Could you check a few things on this drawing? It's one solid part, dimensions in mm from its lowest x, y, z. A direction names the side the tool comes from. Coordinates: 2 decimals unless noted, no trailing zeros. Order: outer loops, then holes, each group sorted by start corner. A loop starts at its lowest first (then second) coordinate and runs counter-clockwise, first axis right, second up.
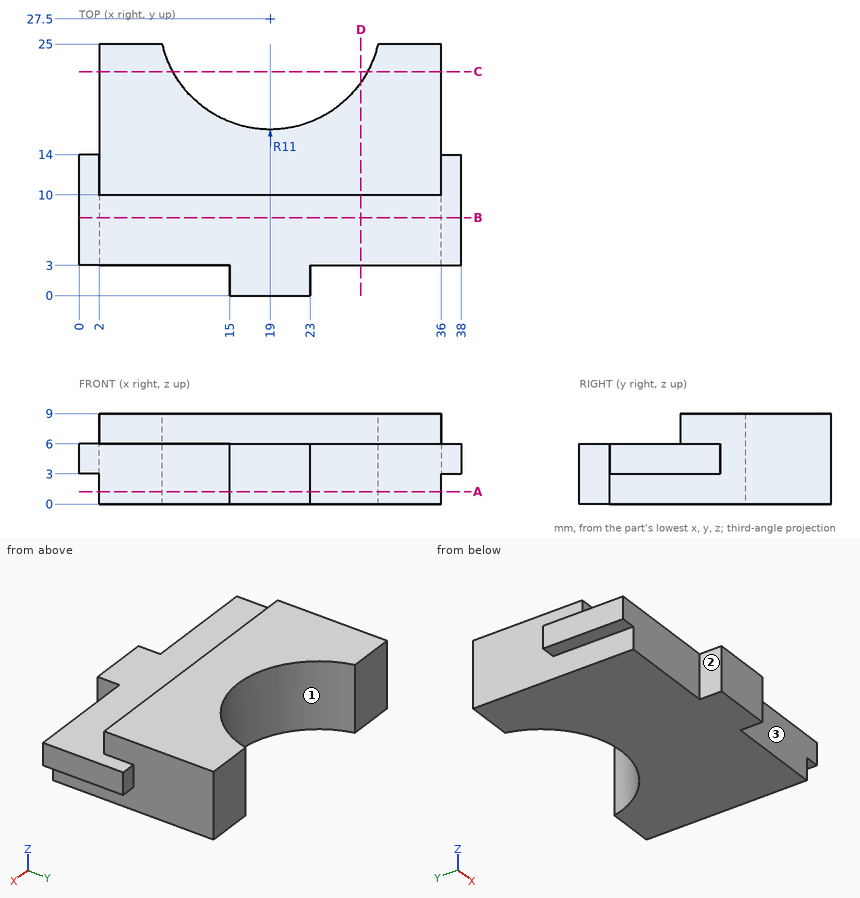
Q1. If we section it at A-A on z = 1.25: Write out the boundary of the cut face in (x, y).
Q2. I need wall thicknesses on L1, parallel to Z at x = 10, y = 5.75; L2, parallel to X at y = 3.25, z = 2.5; L3, parallel to Y at x = 35, z = 8.5. Which ranges of each line are inside material? Lowest first, please.
Q3. If we section it at B-B on y = 7.75: Write out the boundary of the cut face in (x, z), then the cut area to 3 significant figures.
Q4. Will these pins go through, and if not, where does the flat tip stop? pin 1 (5 mm diameter, centred on y = 4, z = 4.5, fed in from -X); pin 2 (5 mm diameter, centred on x = 32.5, z = 3, fed in from -Y); pin 3 (3.5 mm diameter, centred on y = 1, z = 2.5, fed in from +X); pin 4 (1 mm diameter, centred on x = 22.5, y = 3.5, fed in from +Z).
Q5. For the marked faces 1, 2 and 3, which set-ups out of +Z, -Z, +X, -X, +Y, -Y let a thin tool reach every point of the face, with its end or its side?
Q6. If we section it at C-C on y = 22.25: Write out the boundary of the cut face in (x, z), then the cut area to 3 significant figures.
Q7. If we section it at D-D on x = 28: Write out the boundary of the cut face in (y, z).
Reply:
1. outline: (2, 3) - (15, 3) - (15, 0) - (23, 0) - (23, 3) - (36, 3) - (36, 25) - (29.71, 25) arc R11 cw to (8.29, 25) - (2, 25) - close
2. L1: z = 0 to 6
2. L2: x = 2 to 36
2. L3: y = 10 to 25
3. outline: (0, 3) - (2, 3) - (2, 0) - (36, 0) - (36, 3) - (38, 3) - (38, 6) - (0, 6) - close
3. area: 216 mm2
4. pin 1: stops at x = 0
4. pin 2: stops at y = 3
4. pin 3: stops at x = 23
4. pin 4: stops at z = 6
5. face 1: +Z, -Z, +Y
5. face 2: +Z, -Z, -X, -Y
5. face 3: +Z, -Z, +X, -Y
6. outline: (2, 0) - (9.33, 0) - (9.33, 9) - (2, 9) - close; (28.67, 0) - (36, 0) - (36, 9) - (28.67, 9) - close
6. area: 132 mm2
7. outline: (3, 0) - (21.18, 0) - (21.18, 9) - (10, 9) - (10, 6) - (3, 6) - close
